Part model, mm, in its own coordinate system. Face numbers are marked on the shaded views. A direction names the side the tool comes from. Give positions to 0.01 mm unless a question says otherwise; leave off trailing zeros. Loops run counter-clockwise (first coordinate to the right, second up) from the corner with the lowest first, then second, coordinate; pieces in that order, holes last. Notation, with made-up numbers: M 12.25,71 L 51.25,71 A14 ccw 51.25,79 Z; hole C 73.25,50 d9. An arc over 180 degrees is marked long. Put each result on its own line as item: value. Start each with the question number.
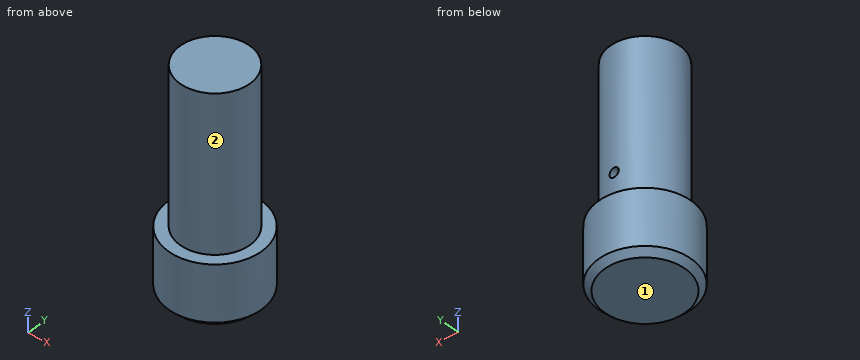
```python
from build123d import *

# Parameters (mm, degrees)
ESQUISSE1_R             = 30
BASE_EXTRUSION_DEPTH    = 40
ESQUISSE2_R             = 22.5
BOSS_EXTRU_1_DEPTH      = 100
ESQUISSE3_R             = 3
ENL_V_MAT_EXTRU_1_DEPTH = 30
CHANFREIN1_SIZE         = 4


with BuildPart() as part:
    # Esquisse1 → Base-Extrusion (new body)
    with BuildSketch(Plane.XY):
        Circle(ESQUISSE1_R)
    extrude(amount=BASE_EXTRUSION_DEPTH)

    # Esquisse2 → Boss.-Extru.1 (add)
    with BuildSketch(Plane.XY.offset(40)):
        Circle(ESQUISSE2_R)
    extrude(amount=BOSS_EXTRU_1_DEPTH)

    # Esquisse3 → Enlèv. mat.-Extru.1 (cut)
    with BuildSketch(Plane(origin=(0, 30, 0), x_dir=(-1, 0, 0), z_dir=(0, 1, 0))):
        with Locations(Location((0, 60, 0), (0, 0, 90))):
            Circle(ESQUISSE3_R)
    extrude(amount=-ENL_V_MAT_EXTRU_1_DEPTH, mode=Mode.SUBTRACT)

    # Chanfrein1
    chanfrein1_edges = [part.edges().sort_by_distance(p)[0] for p in [
        (-30, 0, 0),
    ]]
    chamfer(chanfrein1_edges, length=CHANFREIN1_SIZE)


solid = part.part
```
1) Band-saw the part on A-A on x = 0. Give the cut face in (y, z).
2) Pin check, flat tips, straight feed: pin 1 Ø4 at (x, z) = (-8, 55) entering from +Y; pin 2 Ø5 at (y, z) = (-13.5, 82.5) entering from -X; pin 3 Ø5 at (y, z) = (-14, 115) entering from -X. Stop position of each tip, or through.
3) Wall check: L1, parallel to Z at x = 0, y = 15; L2, parallel to Y at x = 0, z = 39; L3, parallel to X at y = -1, z = 128. Give the ranges that are in metal, low to high.
4) Which spindle directions (+Z, -Z, +X, -X, +Y, -Y) get a long thin tool onto all of the face, cutting with end or side? Do the marked faces 1 and 2. Say none if no direction does.
5) Band-saw the part on B-B on z = 126. Give the cut face in (x, y), then the cut area to 3 significant figures.
6) Band-saw the part on C-C on z = 60. Give the cut face in (x, y).
Evaluation:
1. outline: M -30,4 L -26,0 L 26,0 L 30,4 L 30,40 L 22.5,40 L 22.5,57 L 0,57 L 0,63 L 22.5,63 L 22.5,140 L -22.5,140 L -22.5,40 L -30,40 Z
2. pin 1: y = 21.69
2. pin 2: x = -19.63
2. pin 3: x = -19.34
3. L1: 0 to 57, 63 to 140
3. L2: -30 to 30
3. L3: -22.48 to 22.48
4. face 1: -Z, +X, -X, +Y, -Y
4. face 2: +Z
5. outline: C 0,0 d45
5. area: 1,590 mm2
6. outline: M -3,0 L -3,22.3 A22.5 ccw long 3,22.3 L 3,0 Z
